Answer from the drawing. Dimensions are ordinates in mm from the lowest x, y and z of the part. Coordinates: 2 decimals unless noted, no trailing zeros. Write each loop counter-clockwise with the first axis right and the second up, starting at its lowest first coordinate (ties: lowest second). Pieces come first, ordered by that corner, then holes. Notation, with made-up numbers: (-21, 51) -> (9, 51) arc R9 cw to (9, 65) -> close; hole circle Ø7 at (-23.5, 76.5). An arc over 180 degrees is marked (long way). Answer as a JSON object with one key per item and string values. Group by question number.
(1) Straight lines are drawn through the part: L1, parallel to X at y = 1.8, z = 29; L2, parallel to Z at x = 25.5, y = 2.15; L3, parallel to Z at x = 53, y = 1.05. For each, find the intervals that lie inside material, in ascending order.
(2) Find section A-A (y = 0.75). Give the vertices of the cut face in (x, z) (1 decimal), then the cut area to 3 significant figures.
(3) A flat-ended cylindrical pin translates along its axis: P1, Ø1.5, axis at x = 40.5, y = 1, coming from the +Z side. Find the tip coordinate at first contact, or state that the pin passes through.
(4) Find section C-C (z = 14). Give the vertices of the cut face in (x, y).
(5) Find section B-B (x = 35). Give the vertices of the cut face in (y, z).
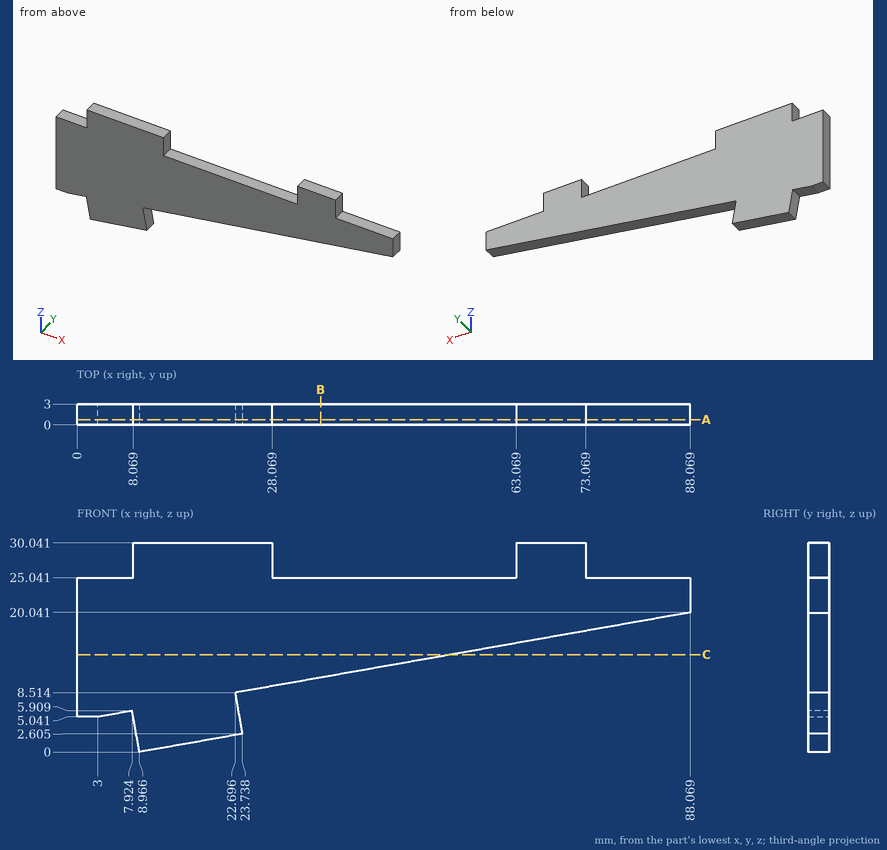
Results below:
{
 "1": {"L1": "x = 8.07 to 28.07, 63.07 to 73.07", "L2": "z = 9.01 to 30.04", "L3": "z = 13.86 to 25.04"},
 "2": {"outline": "(0, 5) -> (3, 5) -> (7.9, 5.9) -> (9, 0) -> (23.7, 2.6) -> (22.7, 8.5) -> (88.1, 20) -> (88.1, 25) -> (73.1, 25) -> (73.1, 30) -> (63.1, 30) -> (63.1, 25) -> (28.1, 25) -> (28.1, 30) -> (8.1, 30) -> (8.1, 25) -> (0, 25) -> close", "area": "1,360 mm2"},
 "3": {"P1": "stops at z = 25.04"},
 "4": {"outline": "(0, 0) -> (53.81, 0) -> (53.81, 3) -> (0, 3) -> close"},
 "5": {"outline": "(0, 10.68) -> (3, 10.68) -> (3, 25.04) -> (0, 25.04) -> close"}
}
